Geometry check sheet. Reference: the model listing, model coordinates, mm. Face numbers are marked on the shaded views. A direction names the side the tool comes from. Coordinates: 2 decimals unless noted, no trailing zeros. Write each loop counter-clockwise with the first axis right and the second up, starting at its lowest first coordinate (ties: lowest second). Pieces come first, ordered by that corner, then holes.
from build123d import *

# Parameters (mm, degrees)
F0_W     = 26.7
F0_H     = 26.7
F1_DEPTH = 6.5
F2_W     = 30
F2_H     = 30
F3_DEPTH = 30
F4_W     = 26.7
F4_H     = 26.7
F5_DEPTH = 13
F6_SIZE  = 5
F7_R     = 10
F8_DEPTH = 56.001


with BuildPart() as f1:
    # F0 (on Front) → F1 (new body, symmetric)
    with BuildSketch(Plane.XZ):
        Rectangle(F0_W, F0_H)
    extrude(amount=F1_DEPTH, both=True)

    # F2 (on face) → F3 (join)
    with BuildSketch(Plane.XZ.offset(6.5)):
        Rectangle(F2_W, F2_H)
    extrude(amount=F3_DEPTH)

    # F4 (on face) → F5 (join)
    with BuildSketch(Plane.XZ.offset(36.5)):
        Rectangle(F4_W, F4_H)
    extrude(amount=F5_DEPTH)

    # F6
    f6_edges = [f1.edges().sort_by_distance(p)[0] for p in [
        (13.35, -43, 13.35),
        (13.35, 0, 13.35),
        (13.35, -43, -13.35),
        (13.35, 0, -13.35),
        (-13.35, -43, 13.35),
        (-13.35, -43, -13.35),
        (-13.35, 0, -13.35),
        (-13.35, 0, 13.35),
        (15, -21.5, 15),
        (-15, -21.5, 15),
        (15, -21.5, -15),
        (-15, -21.5, -15),
    ]]
    chamfer(f6_edges, length=F6_SIZE)

    # F7 (on face) → F8 (cut, through all)
    with BuildSketch(Plane.XZ.offset(49.5)):
        Circle(F7_R)
    extrude(amount=-F8_DEPTH, mode=Mode.SUBTRACT)


solid = f1.part
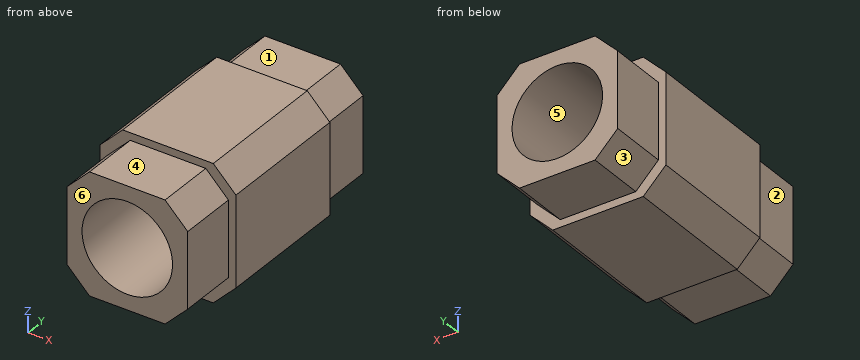
1. Sectioned sample at D-D, the plane x = 10.75. Record the boundary of the cut face in (y, z), and give its area (3 significant figures).
Computed values:
outline: (-49.5, -10.95) - (-36.5, -10.95) - (-36.5, -14.25) - (-6.5, -14.25) - (-6.5, -10.95) - (6.5, -10.95) - (6.5, 10.95) - (-6.5, 10.95) - (-6.5, 14.25) - (-36.5, 14.25) - (-36.5, 10.95) - (-49.5, 10.95) - close
area: 1,420 mm2
2. Gauge pin test, flat ends, axial feed: pin 1 Ø1 at (x, y) = (-11.5, -4) entering from +Z; pin 2 Ø10.5 at (x, y) = (-1, -46) entering from -Z; pin 3 Ø1.5 at (y, z) = (-4.5, 1) entering from -X. Record the tip position at first contact, or that the pin passes through.
Computed values:
pin 1: stops at z = 10.7
pin 2: stops at z = -13.35
pin 3: stops at x = -13.35
3. Thickness scan on line 1 along Z through (x, y) = (0, -29); line 2 along X through (y, z) = (-20.5, -6); line 3 along X through (y, z) = (-39, 4). Record the ranges inside material, lowest first.
Computed values:
line 1: z = -15 to -10, 10 to 15
line 2: x = -15 to -8, 8 to 15
line 3: x = -13.35 to -9.17, 9.17 to 13.35
4. Sectioned sample at B-B, the plane x = 0. Record the boundary of the cut face in (y, z).
Computed values:
outline: (-49.5, -13.35) - (-36.5, -13.35) - (-36.5, -15) - (-6.5, -15) - (-6.5, -13.35) - (6.5, -13.35) - (6.5, -10) - (-49.5, -10) - close; (-49.5, 10) - (6.5, 10) - (6.5, 13.35) - (-6.5, 13.35) - (-6.5, 15) - (-36.5, 15) - (-36.5, 13.35) - (-49.5, 13.35) - close
5. Sectioned sample at C-C, the plane y = -8.5. Record the boundary of the cut face in (x, z).
Computed values:
outline: (-15, -10) - (-10, -15) - (10, -15) - (15, -10) - (15, 10) - (10, 15) - (-10, 15) - (-15, 10) - close; hole circle Ø20 at (0, 0)
6. Access from +Z, -Z, +X, -X, +Y, -Y to the whole of each face (thin tool, end or side, straight path). Record for the marked faces 1, 2 and 3.
Computed values:
face 1: +Z, +X, -X, +Y
face 2: +Z, -Z, -X, -Y
face 3: -Z, -X, +Y
7. Draft check along Z on the marked faces 4, 5 and 6. Enter one of: released by +Z, released by -Z, zero draft, split by the parting line, or undercut.
Computed values:
face 4: released by +Z
face 5: undercut
face 6: zero draft
8. Sectioned sample at A-A, the plane z = 0. Record the boundary of the cut face in (x, y).
Computed values:
outline: (-15, -36.5) - (-13.35, -36.5) - (-13.35, -49.5) - (-10, -49.5) - (-10, 6.5) - (-13.35, 6.5) - (-13.35, -6.5) - (-15, -6.5) - close; (10, -49.5) - (13.35, -49.5) - (13.35, -36.5) - (15, -36.5) - (15, -6.5) - (13.35, -6.5) - (13.35, 6.5) - (10, 6.5) - close
